Can you work these out from the model? Positions are in its coordinate system, mm. A direction names the side the tool comes from. Give positions to 0.01 mm unless a question says otherwise; leave off trailing zeros. Order: outer loops, then holes, each group sorted by start corner. A loop starts at its lowest first (then second) coordinate and runs counter-clockwise, first axis right, second up.
Item 1: Which directions (+Z, -Z, +X, -X, +Y, -Y) give clear straight access to the entire face, cutting with the end or side of a thin tool? Please do faces 4 (the cylindrical face through (35.49, -0.76, 52.69)), 5 (the cylindrical face through (-0.27, 33.28, -52.69)), 6 (the flat face through (6, 31, 57)).
Item 2: I want a section at B-B, the plane z = 19. Write out the boundary of the cut face in (x, y), then the cut area to 3 significant figures.
Item 3: If we mould it in two halves opening along X, with no side actions, what happens to faces 1 (the cylindrical face through (-34.58, -0.89, -35.61)), 2 (the cylindrical face through (8.238, 37.096, 0.798)), 3 (the cylindrical face through (-35.49, -0.76, -52.69))? For each: +X half, -X half, draft (parallel to the pull), parting line (faces both ways), or undercut.
Item 4: I want a section at C-C, the plane y = -13. Write out the boundary of the cut face in (x, z), then the cut area to 3 significant figures.
Item 5: I'm going to push flat-ended pins straight in: pin 1 Ø1.5 at (x, y) = (0, -34.5) entering from +Z; pin 2 Ø2 at (x, y) = (34.5, 0) entering from +Z; pin 3 Ø12 at (y, z) = (16, -2.5) entering from +X. Where does each tip first touch, or does it pass through?
Item 6: I want a section at A-A, the plane y = 20. Write out the boundary of the cut face in (x, z).
Item 7: If I drill on line 1 along Y through (x, z) = (0, -6); line 2 along Y through (x, z) = (0, -52); line 3 along X through (y, z) = (14, -42.5), over which ranges is the centre line in solid material (lowest first)?
```python
from build123d import *

# Parameters (mm, degrees)
SKETCH_1_R                   = 38
SKETCH_1_R_2                 = 31.1
EXTRUDE_1_DEPTH              = 57
HOLE_WIZARD_M3_1_D           = 2.5
HOLE_WIZARD_M3_1_DEPTH       = 8.5
HOLE_WIZARD_M3_1_TIP         = 0.751075774
HOLE_WIZARD_M3_3_D           = 2.5
HOLE_WIZARD_M3_3_DEPTH       = 8.5
HOLE_WIZARD_M3_3_TIP         = 0.751075774
HOLE_WIZARD_M4_1_D           = 3.3
HOLE_WIZARD_M4_1_ON_FACE_2_D = 3.3


with BuildPart() as part:
    # 草图1 → 凸台-拉伸1 (new, symmetric)
    with BuildSketch(Plane.XY):
        with Locations(Location((0, 0, 0), (0, 0, 180))):
            Circle(SKETCH_1_R)
        with Locations(Location((0, 0, 0), (0, 0, 180))):
            Circle(SKETCH_1_R_2, mode=Mode.SUBTRACT)
    extrude(amount=EXTRUDE_1_DEPTH, both=True)

    # M3 螺纹孔1
    with Locations(Plane.XY.offset(57)):
        with Locations((0, 34.5), (34.5, 0), (0, -34.5), (-34.5, 0)):
            Hole(HOLE_WIZARD_M3_1_D / 2, depth=HOLE_WIZARD_M3_1_DEPTH)
            with Locations((0, 0, -(HOLE_WIZARD_M3_1_DEPTH + HOLE_WIZARD_M3_1_TIP / 2))):  # 118° drill point
                Cone(0, HOLE_WIZARD_M3_1_D / 2, HOLE_WIZARD_M3_1_TIP, mode=Mode.SUBTRACT)

    # M3 螺纹孔3
    with Locations(Plane(origin=(13.806274772, 28.987165745, -57), x_dir=(-1, 0, 0), z_dir=(0, 0, -1))):
        with Locations((48.306274772, -28.987165745), (13.806274772, -63.487165745), (-20.693725228, -28.987165745), (13.806274772, 5.512834255)):
            Hole(HOLE_WIZARD_M3_3_D / 2, depth=HOLE_WIZARD_M3_3_DEPTH)
            with Locations((0, 0, -(HOLE_WIZARD_M3_3_DEPTH + HOLE_WIZARD_M3_3_TIP / 2))):  # 118° drill point
                Cone(0, HOLE_WIZARD_M3_3_D / 2, HOLE_WIZARD_M3_3_TIP, mode=Mode.SUBTRACT)

    # M4 螺纹孔1 (through all)
    with Locations(Plane(origin=(38, 0, -37), x_dir=(0, 1, 0), z_dir=(1, 0, 0))):
        with Locations((0, 0)):
            Hole(HOLE_WIZARD_M4_1_D / 2)

    # M4 螺纹孔1 on face 2 (through all)
    with Locations(Plane(origin=(-38, 0, -37), x_dir=(0, 0, -1), z_dir=(-1, 0, 0))):
        with Locations((0, 0)):
            Hole(HOLE_WIZARD_M4_1_ON_FACE_2_D / 2)


solid = part.part
```
Results list:
1. face 4: +Z
1. face 5: -Z
1. face 6: +Z, +X, -X, +Y, -Y
2. outline: circle Ø76 at (0, 0); hole circle Ø62.2 at (0, 0)
2. area: 1,500 mm2
3. face 1: draft
3. face 2: parting line
3. face 3: undercut
4. outline: (-35.71, -57) - (-28.25, -57) - (-28.25, 57) - (-35.71, 57) - close; (28.25, -57) - (35.71, -57) - (35.71, 57) - (28.25, 57) - close
4. area: 1,700 mm2
5. pin 1: stops at z = 48.2
5. pin 2: stops at z = 48.35
5. pin 3: stops at x = 36.66
6. outline: (-32.31, -57) - (-23.82, -57) - (-23.82, 57) - (-32.31, 57) - close; (23.82, -57) - (32.31, -57) - (32.31, 57) - (23.82, 57) - close
7. line 1: y = -38 to -31.1, 31.1 to 38
7. line 2: y = -38 to -35.75, -33.25 to -31.1, 31.1 to 33.25, 35.75 to 38
7. line 3: x = -35.33 to -27.77, 27.77 to 35.33
